Part model, mm, in its own coordinate system. A direction names the side the tool comes from. Give positions to 0.01 mm unless a question says otherwise; leave off trailing zeros. Write each loop counter-clockwise with the first axis right and the second up, starting at its lowest first coordinate (ties: lowest second). Pieces come first, ordered by that corner, then holes.
```python
from build123d import *

# Parameters (mm, degrees)
BOSS_EXTRUDE1_DEPTH            = 10
F_22_5_22_5_DIAMETER_HOLE1_D   = 22.5
CBORE_FOR_M3_SHCS1_D           = 3.2
CBORE_FOR_M3_SHCS1_CBORE_D     = 6.5
CBORE_FOR_M3_SHCS1_CBORE_DEPTH = 3
BOSS_EXTRUDE2_DEPTH            = 10
SKETCH17_W                     = 12
SKETCH17_H                     = 42
BOSS_EXTRUDE3_DEPTH            = 10
M5_CLEARANCE_HOLE1_D           = 5.3
SKETCH20_W                     = 38.1
SKETCH20_H                     = 38.1
BOSS_EXTRUDE4_DEPTH            = 10
M5_CLEARANCE_HOLE2_D           = 5.3
FILLET6_R                      = 4


with BuildPart() as part:
    # Sketch1 → Boss-Extrude1 (new body)
    with BuildSketch(Plane(origin=(0, 0, 0), x_dir=(1, 0, 0), z_dir=(0, 1, 0))):
        Polygon((60, -21), (60, 21), (21, 21), (21, 60), (-21, 60), (-21, 18), (18, 18), (18, -21), align=None)
    extrude(amount=BOSS_EXTRUDE1_DEPTH)

    # Ø22.5 (22.5) Diameter Hole1 (through all)
    with Locations(Plane(origin=(0, 10, 0), x_dir=(1, 0, 0), z_dir=(0, 1, 0))):
        with Locations((0, 39), (39, 0)):
            Hole(F_22_5_22_5_DIAMETER_HOLE1_D / 2)

    # CBORE for M3 SHCS1 (through all)
    with Locations(Plane(origin=(0, 0, 0), x_dir=(-1, 0, 0), z_dir=(0, -1, 0))):
        with Locations((-54.5, 15.5), (-23.5, 15.5), (-23.5, -15.5), (-54.5, -15.5), (-15.5, 54.5), (-15.5, 23.5), (15.5, 23.5), (15.5, 54.5)):
            CounterBoreHole(CBORE_FOR_M3_SHCS1_D / 2, CBORE_FOR_M3_SHCS1_CBORE_D / 2, CBORE_FOR_M3_SHCS1_CBORE_DEPTH)

    # Sketch16 → Boss-Extrude2 (add)
    with BuildSketch(Plane(origin=(0, 10, 0), x_dir=(1, 0, 0), z_dir=(0, 1, 0))):
        Polygon((17.1, 17.1), (-21, 17.1), (-21, 18), (18, 18), (18, -21), (17.1, -21), align=None)
    extrude(amount=-BOSS_EXTRUDE2_DEPTH)

    # Sketch17 → Boss-Extrude3 (add)
    with BuildSketch(Plane(origin=(0, 10, 0), x_dir=(1, 0, 0), z_dir=(0, 1, 0))):
        with Locations((66, 0)):
            Rectangle(SKETCH17_W, SKETCH17_H)
    boss_extrude3 = extrude(amount=-BOSS_EXTRUDE3_DEPTH)

    # M5 Clearance Hole1 (through all)
    with Locations(Plane(origin=(0, 10, 0), x_dir=(1, 0, 0), z_dir=(0, 1, 0))):
        with Locations((67, 16)):
            m5_clearance_hole1 = Hole(M5_CLEARANCE_HOLE1_D / 2)

    # Mirror1: Boss-Extrude3, M5 Clearance Hole1 across plane
    add(boss_extrude3.mirror(Plane(origin=(0, 0, 0), x_dir=(-0.7071067811865477, 0, 0.7071067811865474), z_dir=(0.7071067811865476, 0, 0.7071067811865476))))
    add(m5_clearance_hole1.mirror(Plane(origin=(0, 0, 0), x_dir=(-0.7071067811865477, 0, 0.7071067811865474), z_dir=(0.7071067811865476, 0, 0.7071067811865476))), mode=Mode.SUBTRACT)

    # Sketch20 → Boss-Extrude4 (add)
    with BuildSketch(Plane(origin=(0, 10, 0), x_dir=(1, 0, 0), z_dir=(0, 1, 0))):
        with Locations((-1.95, -1.95)):
            Rectangle(SKETCH20_W, SKETCH20_H)
    extrude(amount=-BOSS_EXTRUDE4_DEPTH)

    # M5 Clearance Hole2 (through all)
    with Locations(Plane(origin=(0, 10, 0), x_dir=(1, 0, 0), z_dir=(0, 1, 0))):
        with Locations((-16, -1), (-1, -16)):
            Hole(M5_CLEARANCE_HOLE2_D / 2)

    # Fillet6
    fillet6_edges = [part.edges().sort_by_distance(p)[0] for p in [
        (72, 5, -21),
        (72, 5, 21),
        (21, 5, -72),
        (-21, 5, -72),
        (21, 5, -21),
        (-21, 5, 21),
    ]]
    fillet(fillet6_edges, radius=FILLET6_R)


solid = part.part
```
1) 3-axis set-ups, long thin cutter, end or side, ignore diameter. For faces 1 (the face through (46, 5, -21)), 2 (the face through (-17.1, 6.55, -54.57)), 3 (the face through (22, 3, 17)): which of +Z, -Z, +X, -X, +Y, -Y reach the whole face in a straight line?
Answers follow:
face 1: -Z, +X, +Y, -Y
face 2: +Y, -Y
face 3: -Y
2) Wall check: L1, parallel to X at y = 7.75, z = -16; L2, parallel to Z at x = 54.5, y = 5; L3, parallel to Z at x = -1, y = 5.5. Give the ranges that are in metal, low to high.
Answers follow:
L1: x = -21 to 21.98, 25.02 to 52.98, 56.02 to 64.35, 69.65 to 72
L2: z = -21 to -17.1, -13.9 to 13.9, 17.1 to 21
L3: z = -72 to -50.21, -27.79 to 13.35, 18.65 to 21
3) Saw through at A-A, the plane x = 54.5. Write the cut outline in (y, z).
Answers follow:
outline: (0, -21) - (10, -21) - (10, -17.1) - (3, -17.1) - (3, -18.75) - (0, -18.75) - close; (0, -12.25) - (3, -12.25) - (3, -13.9) - (10, -13.9) - (10, 13.9) - (3, 13.9) - (3, 12.25) - (0, 12.25) - close; (0, 18.75) - (3, 18.75) - (3, 17.1) - (10, 17.1) - (10, 21) - (0, 21) - close
4) Saw through at C-C, the plane x = 39. Write the cut outline in (y, z).
Answers follow:
outline: (0, -21) - (10, -21) - (10, -11.25) - (0, -11.25) - close; (0, 11.25) - (10, 11.25) - (10, 21) - (0, 21) - close
5) Saw through at B-B, the plane y = 1.25. Count the separate pieces of the cut face and the enclosed holes in it, then the cut area to 3 significant figures.
Answers follow:
separate pieces: 1
enclosed holes: 14
area: 4,890 mm2
6) Pin check, flat tips, straight feed: pin 1 Ø2 at (x, z) = (16, -54) entering from -Y; pin 2 Ø2 at (y, z) = (5, -36) entering from +X. Stop position of each tip, or through.
Answers follow:
pin 1: stops at y = 3
pin 2: stops at x = 21
7) Two-plate mould, pull along X, no slides. Class faces 4 (the face through (70.797, 4.93, 19.859)), 5 (the face through (25.895, 1.479, 13.303)), 6 (the face through (25, 5, 21)): +X half, -X half, draft (parallel to the pull), parting line (faces both ways), or undercut.
Answers follow:
face 4: +X half
face 5: undercut
face 6: draft
8) Saw through at D-D, the plane z = 6. Write the cut outline in (x, y).
Answers follow:
outline: (-21, 0) - (29.48, 0) - (29.48, 10) - (-21, 10) - close; (48.52, 0) - (72, 0) - (72, 10) - (48.52, 10) - close
